Autodesk Inventor part; units mm, degrees
ref_plane "YZ Plane" through (0, 0, 0) normal (1, 0, 0) x (0, 1, 0)
ref_plane "XZ Plane" through (0, 0, 0) normal (0, 1, 0) x (-1, 0, 0)
ref_plane "XY Plane" through (0, 0, 0) normal (0, 0, 1) x (1, 0, 0)
sketch "Sketch1" plane through (0, 0, 0) normal (0, 0, 1) x (1, 0, 0)
  line L0 (-55, 50) -> (55, 50)
  line L1 (55, 50) -> (55, -50)
  line L2 (55, -50) -> (-55, -50)
  line L3 (-55, -50) -> (-55, 50)
  line L4 (41, 36) -> (-41, 36)
  line L5 (-41, 36) -> (-41, -36)
  line L6 (-41, -36) -> (41, -36)
  line L7 (41, -36) -> (41, 36)
  line L8 (0, 152.7233) -> (0, -72.1628) construction
  line L9 (-77.8847, 0) -> (88.8171, 0) construction
  line L10 (-55, 41) -> (55, 41) construction
  circle A0 centre (0, 41) radius 2.25
  circle A1 centre (-19.75, 41) radius 2.25
  circle A2 centre (19.75, 41) radius 2.25
  line L11 (-46, 50) -> (-46, -50) construction
  circle A3 centre (-46, 41) radius 2.25
  circle A4 centre (-46, 0) radius 2.25
  line L12 (-55, -41) -> (55, -41) construction
  circle A5 centre (-46, -41) radius 2.25
  circle A6 centre (-46, 19.75) radius 2.25
  circle A7 centre (-46, -19.75) radius 2.25
  line L13 (0, -20.5) -> (-19.3412, 13) construction
  line L14 (-19.3412, 13) -> (19.3412, 13) construction
  line L15 (19.3412, 13) -> (0, -20.5) construction
  circle A8 centre (19.3412, 13) radius 12.5
  circle A9 centre (-19.3412, 13) radius 12.5
  circle A10 centre (0, -20.5) radius 12.5
  circle A11 centre (-19.3412, 13) radius 20.5
  circle A12 centre (19.3412, 13) radius 20.5
  circle A13 centre (0, -20.5) radius 20.5
  line L16 (-22.8412, 30.0471) -> (-15.8412, 30.0471)
  line L17 (-15.8412, 30.0471) -> (-15.8412, 36)
  line L18 (-15.8412, 36) -> (-22.8412, 36)
  line L19 (-22.8412, 36) -> (-22.8412, 30.0471)
  line L20 (15.8412, 30.0471) -> (22.8412, 30.0471)
  line L21 (22.8412, 30.0471) -> (22.8412, 36)
  line L22 (22.8412, 36) -> (15.8412, 36)
  line L23 (15.8412, 36) -> (15.8412, 30.0471)
  line L24 (-35.3273, 16.5) -> (-41, 16.5)
  line L25 (-41, 16.5) -> (-41, 9.5)
  line L26 (-41, 9.5) -> (-35.3273, 9.5)
  line L27 (-35.3273, 9.5) -> (-35.3273, 16.5)
  line L28 (34.9738, 16.5) -> (41, 16.5)
  line L29 (41, 16.5) -> (41, 9.5)
  line L30 (41, 9.5) -> (34.9738, 9.5)
  line L31 (34.9738, 9.5) -> (34.9738, 16.5)
  line L32 (-3.5, -36.2367) -> (3.5, -36.2367)
  line L33 (3.5, -36.2367) -> (3.5, -36)
  line L34 (3.5, -36) -> (-3.5, -36)
  line L35 (-3.5, -36) -> (-3.5, -36.2367)
  line L36 (-16.3125, -17) -> (-41, -17)
  line L37 (-41, -17) -> (-41, -24)
  line L38 (-41, -24) -> (-16.3125, -24)
  line L39 (-16.3125, -24) -> (-16.3125, -17)
  line L40 (16.0929, -17) -> (41, -17)
  line L41 (41, -17) -> (41, -24)
  line L42 (41, -24) -> (16.0929, -24)
  line L43 (16.0929, -24) -> (16.0929, -17)
  point P0 (0, 0)
  point P1 (0, 50)
  point P2 (55, 0)
  point P3 (0, 1.8333)
  point P4 (-16.3125, -20.5)
  point P5 (16.0929, -20.5)
  point P6 (34.9738, 13)
  point P7 (-35.3273, 13)
  point P8 (-19.3412, 30.0471)
  point P9 (19.3412, 30.0471)
  point P10 (0, -36.2367)
  dimension "d0" = 110
  dimension "d1" = 100
  dimension "d2" = 14
  dimension "d5" = 9
  dimension "d6" = 4.5
  dimension "d7" = 4.5
  dimension "d8" = 4.5
  dimension "d9" = 22
  dimension "d10" = 22
  dimension "d11" = 9
  dimension "d12" = 4.5
  dimension "d13" = 4.5
  dimension "d14" = 9
  dimension "d15" = 4.5
  dimension "d31" = 4.5
  dimension "d32" = 4.5
  dimension "d33" = 22
  dimension "d34" = 22
  dimension "d53" = 23
  dimension "d54" = 25
  dimension "d55" = 25
  dimension "d56" = 25
  dimension "d65" = 8
  dimension "d66" = 8
  dimension "d67" = 8
  dimension "d68" = 7
  dimension "d69" = 7
  dimension "d70" = 7
  dimension "d71" = 7
  dimension "d72" = 7
  dimension "d73" = 7
  dimension "d74" = 7
  dimension "d75" = 38.6825
extrude "Extrusion1" add sketch "Sketch1" along normal blind 1.5 contours L0 L1 L2 L3 | L21 A12 L23 L4 | L7 L30 A12 L28 | L21 L20 L23 A12 | A12 L28 L31 L30 A13 A11 L23 L20 L21 | A12 L30 L31 L28 | L17 A11 L19 L4 | L7 L42 A13 L40 | L17 L16 L19 A11 | A11 A12 A13 L26 L27 L24 L19 L16 L17 | A11 A12 | L40 L43 L42 A13 L6 L38 L39 L36 A11 A12 | A13 L42 L43 L40 | A12 A13 | L24 A11 L26 L5 | L24 L27 L26 A11 | A11 A13 | A13 L6 L35 L32 L33 | L33 L32 L35 L6 | L36 A13 L38 L5 | L36 L39 L38 A13 | A0 | A1 | A2 | A3 | A4 | A5 | A6 | A7
extrude "Extrusion2" cut sketch "Sketch1" along normal blind 10 contours A1 | A2
mirror "Mirror1" about plane through (0, 0, 0) normal (0, 1, 0) of "Extrusion2"
extrude "Extrusion3" cut sketch "Sketch1" along normal blind 10 contours A3 | A5 | A6 | A7
mirror "Mirror2" about plane through (0, 0, 0) normal (1, 0, 0) of "Extrusion3"
extrude "Extrusion7" cut sketch "Sketch1" along normal blind 10 contours L7 L28 A12 L21 L4 | L23 A12 A11 L17 L4 | L7 L40 A13 A12 L30 | L19 A11 L24 L5 L4 | L7 L6 A13 L42 | L40 L43 L42 A13 L6 L38 L39 L36 A11 A12 | A12 A13 A11 | L26 A11 A13 L36 L5 | L6 L5 L38 A13
extrude "Extrusion8" add sketch "Sketch1" along normal blind 1.5 contours L40 L43 L42 A13 L6 L38 L39 L36 A11 A12 | A13 L42 L43 L40 | A12 A13 | A11 A13 | A13 L6 L35 L32 L33 | L36 L39 L38 A13
fillet "Fillet1" radius 15 4 edges at (-55, -50, 0.75) (55, -50, 0.75) (55, 50, 0.75) (-55, 50, 0.75)
properties part number "Base"
Here's how the part is built. I have some questions about the finished solid (model axes, mm). Coordinates: 2 decimals unless noted, no trailing zeros. Loops run counter-clockwise (first coordinate to the right, second up) from the corner with the lowest first, then second, coordinate; pieces in that order, holes last. Notation, with made-up numbers: (-19, -0.75) -> (-15, -0.75) arc R34 ccw to (-15, 37.25) -> close; hole circle Ø8 at (72, -16). An arc over 180 degrees is marked (long way). Use one line per item in the form item = value. Start each with the question number.
(1) If we section it at D-D (y = -2.5): Please give me the cut outline in (x, z).
(2) We'd pull the mould along Y, two halves only. Please class faces 1 (the face through (11, 1, 1.5)), 2 (the face through (-50.49, 45.72, 0.76)), 3 (the face through (-18.54, -42.897, 0.74)), 4 (the face through (-6.22, 28.75, 0.74)): pulls with the +Y half, pulls with the -Y half, needs draft (parallel to the pull), parting line crosses it, or undercut.
(3) If we section it at A-A (x = 45): Please give me the cut outline in (y, z), then the cut area to 3 significant figures.
(4) If we section it at C-C (x = 34): Please give me the cut outline in (y, z).
(5) If we section it at B-B (y = 30): Please give me the cut outline in (x, z).
(6) Please list where these lines run through material, in increasing order: line 1 along X through (y, z) = (33.5, 1.05); line 2 along Y through (x, z) = (-46, 0.4); line 3 along Y through (x, z) = (-8, 1.05).
Verdict:
q1.outline = (-55, 0) -> (-41, 0) -> (-41, 1.5) -> (-55, 1.5) -> close; (-32.76, 0) -> (32.76, 0) -> (32.76, 1.5) -> (-32.76, 1.5) -> close; (41, 0) -> (55, 0) -> (55, 1.5) -> (41, 1.5) -> close
q2.face_1 = needs draft
q2.face_2 = pulls with the +Y half
q2.face_3 = undercut
q2.face_4 = undercut
q3.outline = (-49.14, 0) -> (-43.02, 0) -> (-43.02, 1.5) -> (-49.14, 1.5) -> close; (-38.98, 0) -> (-21.77, 0) -> (-21.77, 1.5) -> (-38.98, 1.5) -> close; (-17.73, 0) -> (17.73, 0) -> (17.73, 1.5) -> (-17.73, 1.5) -> close; (21.77, 0) -> (38.98, 0) -> (38.98, 1.5) -> (21.77, 1.5) -> close; (43.02, 0) -> (49.14, 0) -> (49.14, 1.5) -> (43.02, 1.5) -> close
q3.area = 123 mm²
q4.outline = (-50, 0) -> (-36, 0) -> (-36, 1.5) -> (-50, 1.5) -> close; (-24, 0) -> (-17, 0) -> (-17, 1.5) -> (-24, 1.5) -> close; (-1.33, 0) -> (27.33, 0) -> (27.33, 1.5) -> (-1.33, 1.5) -> close; (36, 0) -> (50, 0) -> (50, 1.5) -> (36, 1.5) -> close
q5.outline = (-55, 0) -> (-41, 0) -> (-41, 1.5) -> (-55, 1.5) -> close; (-30.8, 0) -> (-7.88, 0) -> (-7.88, 1.5) -> (-30.8, 1.5) -> close; (7.88, 0) -> (30.8, 0) -> (30.8, 1.5) -> (7.88, 1.5) -> close; (41, 0) -> (55, 0) -> (55, 1.5) -> (41, 1.5) -> close
q6.line_1 = -55 to -41, -22.84 to -15.84, 15.84 to 22.84, 41 to 55
q6.line_2 = -48.75 to -43.25, -38.75 to -22, -17.5 to 17.5, 22 to 38.75, 43.25 to 48.75
q6.line_3 = -50 to -30.1, -10.9 to 7.74, 18.26 to 30.08, 36 to 50
